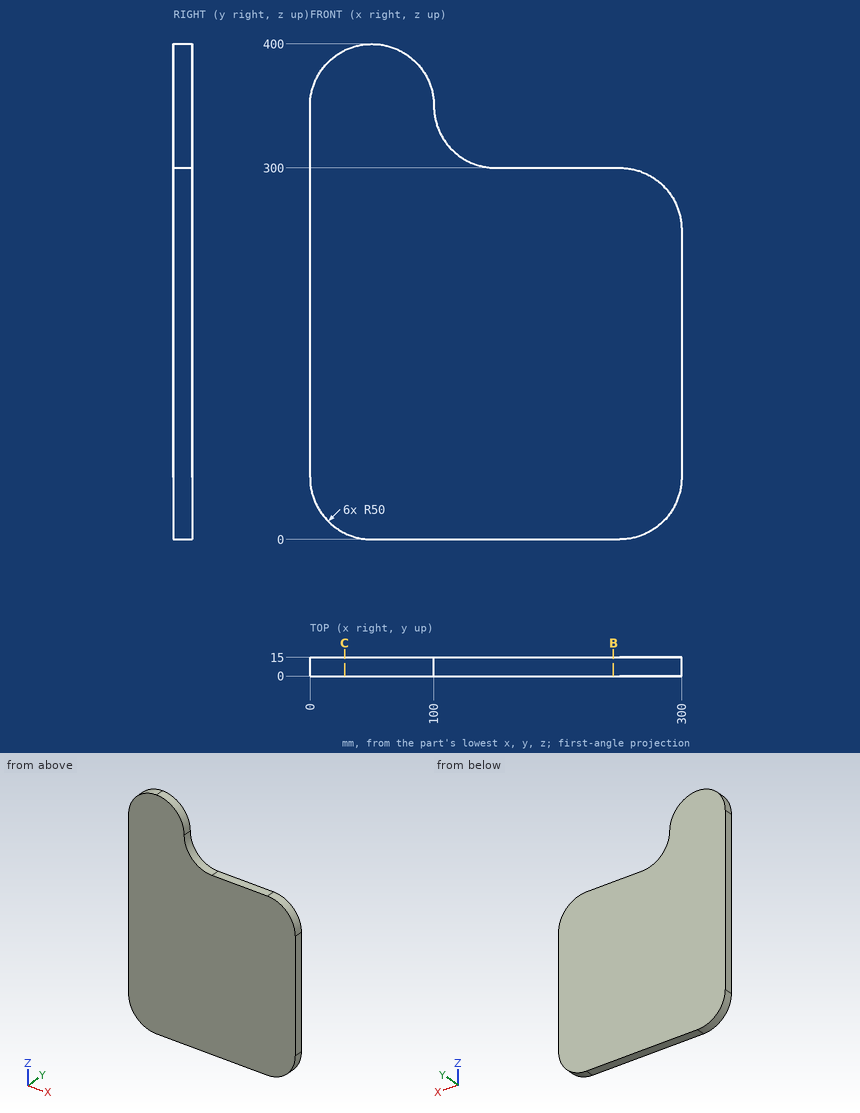
Drawing for the job (mm, zero at the part's lowest x, y, z). Coordinates: 2 decimals unless noted, no trailing zeros. Order: outer loops, then holes, each group sorted by start corner. A loop starts at its lowest first (then second) coordinate and runs counter-clockwise, first axis right, second up. Notation, with made-up numbers: (36, 60) - (74, 60) arc R13 cw to (74, 73) - close; hole circle Ø3 at (9.5, 33.25). An arc over 180 degrees is marked (long way). Use a Markdown table: item, result. Add a question column.
(1) Saw through at C-C (x = 28). Give the cut face in (y, z).
(2) Drill centre lines: line 1 along X through (y, z) = (10, 352.5); line 2 along X through (y, z) = (2, 349); line 3 along Z through (x, y) = (22.5, 8.5). Where is each one in solid material? Low to high. Write a range as [from, to].
(3) Flat gauge pins, fed straight in: pin 1 (6 mm diameter, centred on x = 253, y = 6, fed in from +Z); pin 2 (2 mm diameter, centred on y = 3, z = 344, fed in from -X). Where does each tip first touch, or does it go through?
(4) Saw through at B-B (x = 245). Give the cut face in (y, z), then the cut area to 3 significant figures.
Solved:
| question | item | result |
|---|---|---|
| 1 | outline | (0, 5.1) - (15, 5.1) - (15, 394.9) - (0, 394.9) - close |
| 2 | line 1 | x = [0.06, 99.94] |
| 2 | line 2 | x = [0, 100.01] |
| 2 | line 3 | z = [8.24, 391.76] |
| 3 | pin 1 | stops at z = 300 |
| 3 | pin 2 | stops at x = 0 |
| 4 | outline | (0, 0) - (15, 0) - (15, 300) - (0, 300) - close |
| 4 | area | 4,500 mm² |
